```python
from build123d import *

# Parameters (mm, degrees)
F0_R      = 8
F1_DEPTH  = 10
F2_R      = 16
F3_R      = 8
F4_DEPTH  = 10.001
F6_DEPTH  = 75
F8_DEPTH  = 62.001
F9_R      = 20
F10_DEPTH = 8
F11_R     = 20
F12_DEPTH = 8
F13_R     = 17
F14_DEPTH = 38
F15_R     = 10
F16_DEPTH = 114.001
F17_W     = 12
F17_H     = 10
F18_DEPTH = 75
F19_R     = 10
F20_DEPTH = 132.536
F22_DEPTH = 10


with BuildPart() as f1:
    # F0 (on Front) → F1 (new body)
    with BuildSketch(Plane.XZ):
        with BuildLine():
            Line((59.051879, 108.007187), (-54.948121, 108.007187))
            Line((-54.948121, 108.007187), (-54.948121, 58.007187))
            Line((-54.948121, 58.007187), (-18.163779, -27.671937))
            ThreePointArc((-18.163779, -27.671937), (2.051879, -40.992813), (22.267536, -27.671937))
            Line((22.267536, -27.671937), (59.051879, 58.007187))
            Line((59.051879, 58.007187), (59.051879, 108.007187))
        make_face()
        with Locations((2.051879, -18.992813)):
            Circle(F0_R, mode=Mode.SUBTRACT)
    extrude(amount=F1_DEPTH)

    # F2
    f2_edges = [f1.edges().sort_by_distance(p)[0] for p in [
        (-54.948121, -5, 108.007187),
        (59.051879, -5, 108.007187),
    ]]
    fillet(f2_edges, radius=F2_R)

    # F3 (on face) → F4 (cut, through all)
    with BuildSketch(Plane(origin=(0, 0, 0), x_dir=(-1, 0, 0), z_dir=(0, 1, 0))):
        with Locations((-43.051879, 92.007187)):
            Circle(F3_R)
        with Locations((38.948121, 92.007187)):
            Circle(F3_R)
    extrude(amount=-F4_DEPTH, mode=Mode.SUBTRACT)

    # F5 (on face) → F6 (join)
    with BuildSketch(Plane.XZ.offset(10)):
        Polygon((7.051879, 108.007187), (2.051879, 108.007187), (-2.948121, 108.007187), (-2.948121, 28.007187), (7.051879, 28.007187), align=None)
    extrude(amount=F6_DEPTH)

    # F7 (on face) → F8 (cut, through all)
    with BuildSketch(Plane(origin=(-2.948121, 0, 0), x_dir=(0, -1, 0), z_dir=(-1, 0, 0))):
        with BuildLine():
            Line((85, 108.007187), (10, 108.007187))
            ThreePointArc((10, 108.007187), (11.093214, 104.886516), (13.894876, 103.130274))
            Line((13.894876, 103.130274), (65, 91.542187))
            Line((65, 91.542187), (85, 91.542187))
            Line((85, 91.542187), (85, 108.007187))
        make_face()
        with BuildLine():
            ThreePointArc((13.894876, 32.8841), (11.093214, 31.127858), (10, 28.007187))
            Line((10, 28.007187), (85, 28.007187))
            Line((85, 28.007187), (85, 44.472187))
            Line((85, 44.472187), (65, 44.472187))
            Line((65, 44.472187), (13.894876, 32.8841))
        make_face()
    extrude(amount=-F8_DEPTH, mode=Mode.SUBTRACT)

    # F9 (on face) → F10 (join)
    with BuildSketch(Plane.XY.offset(91.542187)):
        with Locations((2.051879, -85)):
            Circle(F9_R)
    extrude(amount=-F10_DEPTH)

    # F11 (on face) → F12 (join)
    with BuildSketch(Plane(origin=(0, 0, 44.472187), x_dir=(1, 0, 0), z_dir=(0, 0, -1))):
        with Locations((2.051879, 85)):
            Circle(F11_R)
    extrude(amount=-F12_DEPTH)

    # F13 (on face) → F14 (join)
    with BuildSketch(Plane.XY.offset(52.472187)):
        with Locations((2.051879, -85)):
            Circle(F13_R)
    extrude(amount=F14_DEPTH)

    # F15 (on face) → F16 (cut, through all)
    with BuildSketch(Plane.XY.offset(73.007187)):
        with Locations((2.051879, -85)):
            Circle(F15_R)
    extrude(amount=-F16_DEPTH, mode=Mode.SUBTRACT)

    # F17 (on face) → F18 (join)
    with BuildSketch(Plane.XZ.offset(10)):
        Polygon((-43.948121, 73.007187), (-43.948121, 68.007187), (-43.948121, 63.007187), (-14.948121, 63.007187), (-14.948121, 73.007187), align=None)
        with Locations((-8.948121, 68.007187)):
            Rectangle(F17_W, F17_H)
        Polygon((19.051879, 63.007187), (48.051879, 63.007187), (48.051879, 73.007187), (19.051879, 73.007187), (7.051879, 73.007187), (7.051879, 63.007187), align=None)
    extrude(amount=F18_DEPTH)

    # F19 (on face) → F20 (cut, through all)
    with BuildSketch(Plane.XY.offset(91.542187)):
        with Locations((2.051879, -85)):
            Circle(F19_R)
    extrude(amount=-F20_DEPTH, mode=Mode.SUBTRACT)

    # F21 (on face) → F22 (cut)
    with BuildSketch(Plane.XY.offset(73.007187)):
        with BuildLine():
            Line((48.051879, -85), (48.051879, -10))
            ThreePointArc((48.051879, -10), (45.138421, -10.936533), (43.316383, -13.395295))
            Line((43.316383, -13.395295), (19.051879, -85))
            Line((19.051879, -85), (48.051879, -85))
        make_face()
        with BuildLine():
            Line((-43.948121, -85), (-14.948121, -85))
            Line((-14.948121, -85), (-39.212626, -13.395295))
            ThreePointArc((-39.212626, -13.395295), (-41.034663, -10.936533), (-43.948121, -10))
            Line((-43.948121, -10), (-43.948121, -85))
        make_face()
    extrude(amount=-F22_DEPTH, mode=Mode.SUBTRACT)


solid = f1.part
```
Part model, mm, in its own coordinate system. A direction names the side the tool comes from. Round coordinates to 2 decimals unless told otherwise and drop trailing zeros. Write each loop counter-clockwise with the first axis right and the second up, starting at its lowest first coordinate (ties: lowest second). Pieces come first, ordered by that corner, then holes. Notation, with made-up numbers: (53.25, -5.75) -> (65.25, -5.75) arc R23 cw to (65.25, 8.25) -> close; hole circle Ø9 at (51.25, 14). An arc over 180 degrees is marked (long way). Return JSON: item names as keys, results as strings. Group by question number.
Q1. Which spindle directions (+Z, -Z, +X, -X, +Y, -Y) get a long thin tool onto all of the face, cutting with end or side? Do faces 4 (the flat face through (-36.813, -4.93, 15.767)), 5 (the flat face through (-4, -101.3, 83.542)), 6 (the flat face through (-7, -80, 91.542)). Say none if no direction does.
Q2. Mould opens along Y. For faces 1 (the cylindrical face through (-37.2, -4.9, 84.2)), 2 (the flat face through (-19, -39, 73.007)), 3 (the flat face through (1.98, -39.81, 38.76)) say: pulls with the +Y half, pulls with the -Y half, needs draft (parallel to the pull), parting line crosses it, or undercut.
Q3. Saw through at D-D on y = -55. Write the cut outline in (x, z).
Q4. Saw through at C-C on z = 41. Write the cut outline in (x, y), plus the area to 3 significant figures.
Q5. Saw through at B-B on z = 69. Write the cut outline in (x, y), plus the area to 3 significant figures.
Q6. Probe L1, parallel to Y at x = 8, z = 59.5; L2, parallel to Y at x = -26, z = -6.5; L3, parallel to Z at x = 14, y = -26. List the from-to ranges inside material, lowest first. Write a range as [from, to].
Q7. Pin check, flat tips, straight feed: pin 1 (10.5 mm diameter, centred on y = -45.5, z = 84.5, fed in from -X); pin 2 (12 mm diameter, centred on x = -1, y = -77, fed in from -Z); pin 3 (8 mm diameter, centred on x = -28, z = -8.5, fed in from -Y). Stop position of each tip, or through.
Q8. Saw through at A-A on y = -79. Write the cut outline in (x, z).
Answer:
{
 "1": {"face 4": "-Z, -X, +Y, -Y", "face 5": "none", "face 6": "+Z, +X, -X, -Y"},
 "2": {"face 1": "needs draft", "face 2": "undercut", "face 3": "pulls with the -Y half"},
 "3": {"outline": "(-25.11, 63.01) -> (-2.95, 63.01) -> (-2.95, 42.2) -> (7.05, 42.2) -> (7.05, 63.01) -> (29.22, 63.01) -> (29.22, 73.01) -> (7.05, 73.01) -> (7.05, 93.81) -> (-2.95, 93.81) -> (-2.95, 73.01) -> (-25.11, 73.01) -> close"},
 "4": {"outline": "(-47.65, -10) -> (-2.95, -10) -> (-2.95, -49.69) -> (7.05, -49.69) -> (7.05, -10) -> (51.75, -10) -> (51.75, 0) -> (-47.65, 0) -> close", "area": "1,390 mm2"},
 "5": {"outline": "(-54.95, -10) -> (-43.95, -10) arc R5 cw to (-39.21, -13.4) -> (-14.95, -85) arc R17 ccw to (19.05, -85) -> (43.32, -13.4) arc R5 cw to (48.05, -10) -> (59.05, -10) -> (59.05, 0) -> (-54.95, 0) -> close; hole circle Ø20 at (2.05, -85)", "area": "5,740 mm2"},
 "6": {"L1": "[-100.93, -93.04], [-76.96, -69.07], [-10, 0]", "L2": "[-10, 0]", "L3": "[63.01, 73.01]"},
 "7": {"pin 1": "x = -2.95", "pin 2": "z = 44.47", "pin 3": "y = -10"},
 "8": {"outline": "(-17.03, 44.47) -> (-5.95, 44.47) -> (-5.95, 91.54) -> (-17.03, 91.54) -> (-17.03, 83.54) -> (-13.85, 83.54) -> (-13.85, 73.01) -> (-16.98, 73.01) -> (-16.98, 63.01) -> (-13.85, 63.01) -> (-13.85, 52.47) -> (-17.03, 52.47) -> close; (10.05, 44.47) -> (21.13, 44.47) -> (21.13, 52.47) -> (17.96, 52.47) -> (17.96, 63.01) -> (21.09, 63.01) -> (21.09, 73.01) -> (17.96, 73.01) -> (17.96, 83.54) -> (21.13, 83.54) -> (21.13, 91.54) -> (10.05, 91.54) -> close"}
}
